from build123d import *

# Parameters (mm, degrees)
SKETCH1_R           = 8
SKETCH1_R_2         = 4
BOSS_EXTRUDE1_DEPTH = 4.5
CHAMFER1_SIZE       = 0.5
SKETCH2_R           = 7
SKETCH2_R_2         = 5
CUT_EXTRUDE1_DEPTH  = 0.5
SKETCH3_R           = 7
SKETCH3_R_2         = 5
CUT_EXTRUDE2_DEPTH  = 0.5


with BuildPart() as part:
    # Sketch1 → Boss-Extrude1 (new body)
    with BuildSketch(Plane.XY):
        Circle(SKETCH1_R)
        Circle(SKETCH1_R_2, mode=Mode.SUBTRACT)
    extrude(amount=BOSS_EXTRUDE1_DEPTH)

    # Chamfer1
    chamfer1_edges = [part.edges().sort_by_distance(p)[0] for p in [
        (-8, 0, 0),
        (-8, 0, 4.5),
        (-4, 0, 0),
        (-4, 0, 4.5),
    ]]
    chamfer(chamfer1_edges, length=CHAMFER1_SIZE)

    # Sketch2 → Cut-Extrude1 (cut)
    with BuildSketch(Plane.XY):
        Circle(SKETCH2_R)
        Circle(SKETCH2_R_2, mode=Mode.SUBTRACT)
    extrude(amount=CUT_EXTRUDE1_DEPTH, mode=Mode.SUBTRACT)

    # Sketch3 → Cut-Extrude2 (cut)
    with BuildSketch(Plane.XY.offset(4.5)):
        Circle(SKETCH3_R)
        Circle(SKETCH3_R_2, mode=Mode.SUBTRACT)
    extrude(amount=-CUT_EXTRUDE2_DEPTH, mode=Mode.SUBTRACT)


solid = part.part
Check sheet for the modelled part. Datum: model origin and axes. Units: mm. A direction names the side the tool comes from. Round coordinates to 2 decimals unless told otherwise and drop trailing zeros. Order: outer loops, then holes, each group sorted by start corner. A loop starts at its lowest first (then second) coordinate and runs counter-clockwise, first axis right, second up.
Q1. Scan lines: L1, parallel to Y at x = 0, z = 4.25; L2, parallel to Y at x = 0, z = 0.15; L3, parallel to Y at x = 0.5, z = 3.55. Record each from-to range of solid material in increasing order.
Filled sheet:
L1: y = -7.75 to -7, -5 to -4.25, 4.25 to 5, 7 to 7.75
L2: y = -7.65 to -7, -5 to -4.35, 4.35 to 5, 7 to 7.65
L3: y = -7.98 to -3.97, 3.97 to 7.98
Q2. Cross-section at C-C, the plane z = 3.6. Enter the section's corners in (x, y), plus the area to 3 significant figures.
Filled sheet:
outline: circle Ø16 at (0, 0); hole circle Ø8 at (0, 0)
area: 151 mm2
Q3. Set-up check for faces 1 (the face through (7, 2, 4.5)), 2 (the face through (-1.08, -4.88, 4.25)), 3 (the face through (-1.08, -4.88, 0.25)): record each of +Z, -Z, +X, -X, +Y, -Y from which the full face is reachable in a straight line by a thin tool's end or side.
Filled sheet:
face 1: +Z, +X, -X, +Y, -Y
face 2: +Z
face 3: -Z
Q4. Depth check by flat-ended pin: P1, Ø2, axis at x = 3, z = 3.5, coming from the -Y side; P2, Ø1.5, axis at y = 3, z = 2.5, coming from the +X side; P3, Ø1, axis at y = 3, z = 1.5, coming from the +X side. Enter the tip coordinate at first touch or a pass-through.
Filled sheet:
P1: stops at y = -7.75
P2: stops at x = 7.68
P3: stops at x = 7.6
Q5. Draft check along Y on faces 4 (the face through (6.466, -2.681, 4.254)), 5 (the face through (-1.73, -7.81, 2.23)), 6 (the face through (7, 2, 0)). Enter one of: pulls with the +Y half, pulls with the -Y half, needs draft (parallel to the pull), parting line crosses it, or undercut.
Filled sheet:
face 4: undercut
face 5: parting line crosses it
face 6: needs draft
